Could you check a few things on this model? Use its own coordinates, in mm. Face numbers are marked on the shaded views. A direction names the side the tool comes from. Round coordinates to 2 decimals unless told otherwise and drop trailing zeros. Order: outer loops, then holes, each group sorted by start corner. A loop starts at its lowest first (then second) coordinate and runs counter-clockwise, first axis right, second up. Notation, with made-up numbers: M 27.5,44.5 L 70.5,44.5 A24 cw 70.5,70.5 Z; hole C 79,31 d6. An arc over 180 degrees is marked long. Write each question's results on one line, items separated by ' | '. Start each with the question number.
1. I'm going to push flat-ended pins straight in: pin 1 (1.5 mm diameter, centred on x = 2.5, y = 0.5, fed in from -Z); pin 2 (3 mm diameter, centred on y = 0, z = 21.5, fed in from +X); pin 3 (7 mm diameter, centred on y = -1.5, z = 17, fed in from -X); pin 4 (1.8 mm diameter, centred on x = 5.66, y = -5.66, fed in from +Z). Where does each tip first touch, or does it pass through?
2. Suppose I cut it at B-B on y = 8. Write out the boundary of the cut face in (x, z), and give its area (3 significant figures).
3. For the marked faces 1, 2 and 3, which set-ups out of +Z, -Z, +X, -X, +Y, -Y let a thin tool reach every point of the face, with its end or its side?
4. Suppose I cut it at C-C on y = -6. Write out the boundary of the cut face in (x, z).
5. Suppose I cut it at D-D on z = 37. Write out the boundary of the cut face in (x, y).
6. Please list where these lines run through material, in increasing order: L1, parallel to X at y = 8, z = 3.2; L2, parallel to Z at x = 6.5, y = -1; L3, parallel to Z at x = -1.75, y = -1.25.
7. Suppose I cut it at A-A on x = 0. Write out the boundary of the cut face in (y, z), and give its area (3 significant figures).
Autodesk Inventor part; units mm, degrees
ref_plane "Plano de trabajo1" through (0, 11, 0) normal (0, 1, 0) x (-1, 0, 0)
ref_plane "Plano de trabajo2" through (-11, 0, 0) normal (1, 0, 0) x (0, 1, 0)
ref_plane "XY Plane" through (0, 0, 0) normal (0, 0, 1) x (1, 0, 0)
sketch "Boceto1" plane through (0, 0, 0) normal (0, 0, 1) x (1, 0, 0)
  circle A0 centre (0, 0) radius 11
  dimension "d0" = 22
extrude "Extrusión1" add sketch "Boceto1" along normal blind 4
sketch "Boceto2" plane through (0, 0, 4) normal (0, 0, 1) x (1, 0, 0)
  line L0 (0, 0) -> (0, 8)
  circle A0 centre (0, 8) radius 1
  dimension "d3" = 8
  dimension "d4" = 2
hole "Agujero1" at (0, 8, 4) direction (0, 0, -1) diameter 2.013 end through all
pattern_circular "Patrón circular1" count 8 over 360 about axis through (0, 0, 0) along (0, 0, 1) of "Agujero1"
sketch "Boceto3" plane through (0, 0, 0) normal (0, 0, -1) x (-1, 0, 0)
  circle A0 centre (0, 0) radius 4.4
  dimension "d15" = 8.8
extrude "Extrusión2" cut sketch "Boceto3" against normal blind 2.9
sketch "Boceto4" plane through (0, 0, 2.9) normal (0, 0, -1) x (-1, 0, 0)
  circle A0 centre (0, 0) radius 2.5
  dimension "d18" = 5
extrude "Extrusión3" cut sketch "Boceto4" against normal blind 2.6
sketch "Boceto5" plane through (0, 0, 4) normal (0, 0, 1) x (1, 0, 0)
  circle A0 centre (0, 0) radius 5
  dimension "d21" = 10
extrude "Extrusión4" add sketch "Boceto5" along normal blind 4
sketch "Boceto6" plane through (0, 0, 8) normal (0, 0, 1) x (1, 0, 0)
  arc A0 (-1.9, -3.2909) -> (-1.9, 3.2909) centre (0, 0) ccw
  line L0 (0, 0) -> (-1.9, 0)
  line L1 (-1.9, 0) -> (-1.9, 3.2909)
  line L2 (-1.9, 0) -> (-1.9, -3.2909)
  dimension "DiametroEje" = 7.6
  dimension "d26" = 1.9
extrude "Extrusión5" add sketch "Boceto6" along normal blind 34
ref_plane "Plano de trabajo1" through (0, 11, 0) normal (0, 1, 0) x (-1, 0, 0)
ref_plane "Plano de trabajo2" through (-11, 0, 0) normal (1, 0, 0) x (0, 1, 0)
sketch "Boceto8" plane through (-11, 0, 0) normal (1, 0, 0) x (0, 1, 0)
  line L0 (-1.25, 0) -> (1.25, 0)
  line L1 (1.25, 0) -> (1.25, 4)
  line L2 (1.25, 4) -> (-1.25, 4)
  line L3 (-1.25, 4) -> (-1.25, 0)
  line L4 (-1.25, 0) -> (1.25, 4) construction
  line L5 (1.25, 0) -> (-1.25, 4) construction
  point P0 (0, 0)
  point P1 (0, 2)
  dimension "d33" = 2.5
  dimension "d34" = 4
extrude "Extrusión7" cut sketch "Boceto8" along normal blind 0.5
equation "\"d26\" = 0.25 * DiametroEje"
properties part number "BM-MX28" material "PETG"
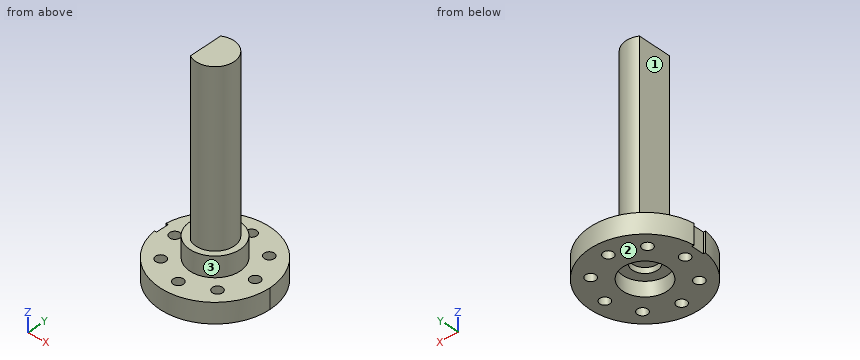
Filled sheet:
1) pin 1: stops at z = 2.9 | pin 2: stops at x = 3.8 | pin 3: stops at x = -1.9 | pin 4: passes through
2) outline: M -7.55,0 L -1.01,0 L -1.01,4 L -7.55,4 Z; M 1.01,0 L 7.55,0 L 7.55,4 L 1.01,4 Z | area: 52.3 mm^2
3) face 1: +Z, -X, +Y, -Y | face 2: -Z, +X, -X, +Y, -Y | face 3: +Z
4) outline: M -9.22,0 L -6.6,0 L -6.6,4 L -9.22,4 Z; M -4.71,0 L 4.71,0 L 4.71,4 L -4.71,4 Z; M 6.6,0 L 9.22,0 L 9.22,4 L 6.6,4 Z
5) outline: M -1.9,-3.29 A3.8 ccw long -1.9,3.29 Z
6) L1: x = -7.55 to -1.01, 1.01 to 7.55 | L2: z = 0 to 4 | L3: z = 4 to 42
7) outline: M -11,0 L -9.01,0 L -9.01,4 L -11,4 Z; M -6.99,0 L -4.4,0 L -4.4,2.9 L -2.5,2.9 L -2.5,4 L 2.5,4 L 2.5,2.9 L 4.4,2.9 L 4.4,0 L 6.99,0 L 6.99,4 L 5,4 L 5,8 L 3.8,8 L 3.8,42 L -3.8,42 L -3.8,8 L -5,8 L -5,4 L -6.99,4 Z; M 9.01,0 L 11,0 L 11,4 L 9.01,4 Z | area: 339 mm^2
